Work out the finished part from the listing and answer in its coordinate system (mm). Face numbers are marked on the shaded views. A direction names the side the tool comes from. Round coordinates to 2 decimals unless told otherwise and drop trailing zeros. Write each loop counter-clockwise with the first axis right and the second up, starting at its lowest first coordinate (ties: lowest second). Pieces come first, ordered by that corner, then holes. Notation, with made-up numbers: M 86.5,35 L 125.5,35 A21 cw 125.5,70 Z; hole C -37,-33 d1. An arc over 180 degrees is marked long. Answer in a Markdown table with one row per item.
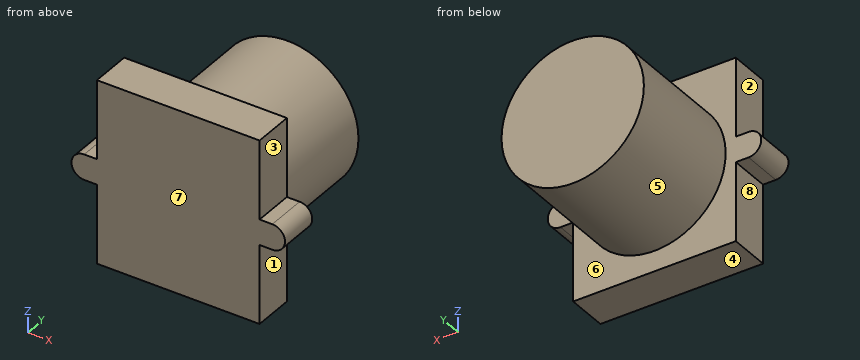
```python
from build123d import *

# Parameters (mm, degrees)
BOSS_EXTRUDE1_DEPTH = 4
SKETCH2_R           = 7
BOSS_EXTRUDE2_DEPTH = 12


with BuildPart() as part:
    # Sketch1 → Boss-Extrude1 (new body)
    with BuildSketch(Plane(origin=(0, 0, 0), x_dir=(1, 0, 0), z_dir=(0, 1, 0))):
        with BuildLine():
            Line((0, 0), (16, 0))
            Line((16, 0), (16, 7.75))
            Line((16, 7.75), (17.25, 7.75))
            ThreePointArc((17.25, 7.75), (18.5, 9), (17.25, 10.25))
            Line((17.25, 10.25), (16, 10.25))
            Line((16, 10.25), (16, 18))
            Line((16, 18), (0, 18))
            Line((0, 18), (0, 10.25))
            Line((0, 10.25), (-1.25, 10.25))
            ThreePointArc((-1.25, 10.25), (-2.5, 9), (-1.25, 7.75))
            Line((-1.25, 7.75), (0, 7.75))
            Line((0, 7.75), (0, 0))
        make_face()
    extrude(amount=BOSS_EXTRUDE1_DEPTH)

    # Sketch2 → Boss-Extrude2 (add)
    with BuildSketch(Plane(origin=(0, 4, 0), x_dir=(1, 0, 0), z_dir=(0, 1, 0))):
        with Locations((8, 9)):
            Circle(SKETCH2_R)
    extrude(amount=BOSS_EXTRUDE2_DEPTH)


solid = part.part
```
1. Given pin 1 (5 mm diameter, centred on y = 11.5, z = -8, fed in from +X); pin 2 (1 mm diameter, centred on y = 7, z = -6, fed in from +X); pin 3 (6 mm diameter, centred on y = 3, z = -3, fed in from +X), each flat-ended and moving along its own axis, determine where each tip first touches the part or whether it passes through.
Calculated:
| item | result |
|---|---|
| pin 1 | stops at x = 15 |
| pin 2 | stops at x = 14.54 |
| pin 3 | stops at x = 16 |
2. The part is cut by section C-C (y = 10.25). Determine the outline of the cut face in (x, z), plus the area to 3 significant figures.
Calculated:
| item | result |
|---|---|
| outline | C 8,-9 d14 |
| area | 154 mm² |
3. A tool of negligible diameter and unlimited length cuts with its end or side. For the marked faces 1, 2, 3, 4 and 5, from which of +Z, -Z, +X, -X, +Y, -Y can it reach the whole face along a straight path? Write none if from no direction.
Calculated:
| item | result |
|---|---|
| face 1 | -Z, +X, +Y, -Y |
| face 2 | +Z, -X, +Y, -Y |
| face 3 | +Z, +X, +Y, -Y |
| face 4 | -Z, +X, -X, +Y, -Y |
| face 5 | +Y |
4. Determine the mould class of the marked faces 6, 7 and 8 for opening direction Y: released by +Y, released by -Y, zero draft, split by the parting line, or undercut.
Calculated:
| item | result |
|---|---|
| face 6 | released by +Y |
| face 7 | released by -Y |
| face 8 | zero draft |
5. The part is cut by section B-B (x = 8). Determine the outline of the cut face in (y, z), plus the area to 3 significant figures.
Calculated:
| item | result |
|---|---|
| outline | M 0,-18 L 4,-18 L 4,-16 L 16,-16 L 16,-2 L 4,-2 L 4,0 L 0,0 Z |
| area | 240 mm² |
6. Consider line 1 along X through (y, z) = (1.25, -2.5); line 2 along Y through (x, z) = (10.75, -16.25); line 3 along Z through (x, y) = (8.5, 12.25). Determine where each line is inside the solid, lowest interval first. Write a range as from..to.
Calculated:
| item | result |
|---|---|
| line 1 | x = 0..16 |
| line 2 | y = 0..4 |
| line 3 | z = -15.98..-2.02 |
7. The part is cut by section D-D (z = -16.5). Determine the outline of the cut face in (x, y).
Calculated:
| item | result |
|---|---|
| outline | M 0,0 L 16,0 L 16,4 L 0,4 Z |
8. The part is cut by section A-A (z = -9). Determine the outline of the cut face in (x, y).
Calculated:
| item | result |
|---|---|
| outline | M -2.5,0 L 18.5,0 L 18.5,4 L 15,4 L 15,16 L 1,16 L 1,4 L -2.5,4 Z |
